```python
from build123d import *

# Parameters (mm, degrees)
F0_W     = 177.8
F0_H     = 137.16
F0_R     = 6.35
F1_DEPTH = 6.35


with BuildPart() as f1:
    # F0 (on Top) → F1 (new body)
    with BuildSketch(Plane.XY):
        with Locations((80.01, 53.34)):
            Rectangle(F0_W, F0_H)
        Circle(F0_R, mode=Mode.SUBTRACT)
        with Locations((17.78, 0)):
            Circle(F0_R, mode=Mode.SUBTRACT)
        with Locations((0, 15.24)):
            Circle(F0_R, mode=Mode.SUBTRACT)
        with Locations((17.78, 15.24)):
            Circle(F0_R, mode=Mode.SUBTRACT)
        with Locations((35.56, 0)):
            Circle(F0_R, mode=Mode.SUBTRACT)
        with Locations((53.34, 0)):
            Circle(F0_R, mode=Mode.SUBTRACT)
        with Locations((71.12, 0)):
            Circle(F0_R, mode=Mode.SUBTRACT)
        with Locations((35.56, 15.24)):
            Circle(F0_R, mode=Mode.SUBTRACT)
        with Locations((53.34, 15.24)):
            Circle(F0_R, mode=Mode.SUBTRACT)
        with Locations((71.12, 15.24)):
            Circle(F0_R, mode=Mode.SUBTRACT)
        with Locations((0, 30.48)):
            Circle(F0_R, mode=Mode.SUBTRACT)
        with Locations((17.78, 30.48)):
            Circle(F0_R, mode=Mode.SUBTRACT)
        with Locations((0, 45.72)):
            Circle(F0_R, mode=Mode.SUBTRACT)
        with Locations((17.78, 45.72)):
            Circle(F0_R, mode=Mode.SUBTRACT)
        with Locations((35.56, 30.48)):
            Circle(F0_R, mode=Mode.SUBTRACT)
        with Locations((53.34, 30.48)):
            Circle(F0_R, mode=Mode.SUBTRACT)
        with Locations((71.12, 30.48)):
            Circle(F0_R, mode=Mode.SUBTRACT)
        with Locations((35.56, 45.72)):
            Circle(F0_R, mode=Mode.SUBTRACT)
        with Locations((53.34, 45.72)):
            Circle(F0_R, mode=Mode.SUBTRACT)
        with Locations((71.12, 45.72)):
            Circle(F0_R, mode=Mode.SUBTRACT)
        with Locations((88.9, 0)):
            Circle(F0_R, mode=Mode.SUBTRACT)
        with Locations((106.68, 0)):
            Circle(F0_R, mode=Mode.SUBTRACT)
        with Locations((124.46, 0)):
            Circle(F0_R, mode=Mode.SUBTRACT)
        with Locations((88.9, 15.24)):
            Circle(F0_R, mode=Mode.SUBTRACT)
        with Locations((106.68, 15.24)):
            Circle(F0_R, mode=Mode.SUBTRACT)
        with Locations((124.46, 15.24)):
            Circle(F0_R, mode=Mode.SUBTRACT)
        with Locations((142.24, 0)):
            Circle(F0_R, mode=Mode.SUBTRACT)
        with Locations((160.02, 0)):
            Circle(F0_R, mode=Mode.SUBTRACT)
        with Locations((142.24, 15.24)):
            Circle(F0_R, mode=Mode.SUBTRACT)
        with Locations((160.02, 15.24)):
            Circle(F0_R, mode=Mode.SUBTRACT)
        with Locations((88.9, 30.48)):
            Circle(F0_R, mode=Mode.SUBTRACT)
        with Locations((106.68, 30.48)):
            Circle(F0_R, mode=Mode.SUBTRACT)
        with Locations((124.46, 30.48)):
            Circle(F0_R, mode=Mode.SUBTRACT)
        with Locations((88.9, 45.72)):
            Circle(F0_R, mode=Mode.SUBTRACT)
        with Locations((106.68, 45.72)):
            Circle(F0_R, mode=Mode.SUBTRACT)
        with Locations((124.46, 45.72)):
            Circle(F0_R, mode=Mode.SUBTRACT)
        with Locations((142.24, 30.48)):
            Circle(F0_R, mode=Mode.SUBTRACT)
        with Locations((160.02, 30.48)):
            Circle(F0_R, mode=Mode.SUBTRACT)
        with Locations((142.24, 45.72)):
            Circle(F0_R, mode=Mode.SUBTRACT)
        with Locations((160.02, 45.72)):
            Circle(F0_R, mode=Mode.SUBTRACT)
        with Locations((0, 60.96)):
            Circle(F0_R, mode=Mode.SUBTRACT)
        with Locations((17.78, 60.96)):
            Circle(F0_R, mode=Mode.SUBTRACT)
        with Locations((35.56, 60.96)):
            Circle(F0_R, mode=Mode.SUBTRACT)
        with Locations((53.34, 60.96)):
            Circle(F0_R, mode=Mode.SUBTRACT)
        with Locations((71.12, 60.96)):
            Circle(F0_R, mode=Mode.SUBTRACT)
        with BuildLine():
            ThreePointArc((8.255, 102.87), (10.114872, 107.360128), (14.605, 109.22))
            Line((14.605, 109.22), (62.865, 109.22))
            ThreePointArc((62.865, 109.22), (67.355128, 107.360128), (69.215, 102.87))
            Line((69.215, 102.87), (69.215, 85.09))
            ThreePointArc((69.215, 85.09), (67.355128, 80.599872), (62.865, 78.74))
            Line((62.865, 78.74), (14.605, 78.74))
            ThreePointArc((14.605, 78.74), (10.114872, 80.599872), (8.255, 85.09))
            Line((8.255, 85.09), (8.255, 102.87))
        make_face(mode=Mode.SUBTRACT)
        with Locations((88.9, 60.96)):
            Circle(F0_R, mode=Mode.SUBTRACT)
        with Locations((106.68, 60.96)):
            Circle(F0_R, mode=Mode.SUBTRACT)
        with Locations((124.46, 60.96)):
            Circle(F0_R, mode=Mode.SUBTRACT)
        with Locations((88.9, 76.2)):
            Circle(F0_R, mode=Mode.SUBTRACT)
        with Locations((106.68, 76.2)):
            Circle(F0_R, mode=Mode.SUBTRACT)
        with Locations((124.46, 76.2)):
            Circle(F0_R, mode=Mode.SUBTRACT)
        with Locations((142.24, 60.96)):
            Circle(F0_R, mode=Mode.SUBTRACT)
        with Locations((160.02, 60.96)):
            Circle(F0_R, mode=Mode.SUBTRACT)
        with Locations((142.24, 76.2)):
            Circle(F0_R, mode=Mode.SUBTRACT)
        with Locations((160.02, 76.2)):
            Circle(F0_R, mode=Mode.SUBTRACT)
        with Locations((88.9, 91.44)):
            Circle(F0_R, mode=Mode.SUBTRACT)
        with Locations((106.68, 91.44)):
            Circle(F0_R, mode=Mode.SUBTRACT)
        with Locations((124.46, 91.44)):
            Circle(F0_R, mode=Mode.SUBTRACT)
        with Locations((88.9, 106.68)):
            Circle(F0_R, mode=Mode.SUBTRACT)
        with Locations((106.68, 106.68)):
            Circle(F0_R, mode=Mode.SUBTRACT)
        with Locations((124.46, 106.68)):
            Circle(F0_R, mode=Mode.SUBTRACT)
        with Locations((142.24, 91.44)):
            Circle(F0_R, mode=Mode.SUBTRACT)
        with Locations((160.02, 91.44)):
            Circle(F0_R, mode=Mode.SUBTRACT)
        with Locations((142.24, 106.68)):
            Circle(F0_R, mode=Mode.SUBTRACT)
        with Locations((160.02, 106.68)):
            Circle(F0_R, mode=Mode.SUBTRACT)
    extrude(amount=F1_DEPTH)


solid = f1.part
```
Build history of the part. All positions in model axes, mm. Round coordinates to 2 decimals unless told otherwise and drop trailing zeros. Order: outer loops, then holes, each group sorted by start corner. A loop starts at its lowest first (then second) coordinate and runs counter-clockwise, first axis right, second up. Notation, with made-up numbers: (70, -34.5) -> (113, -34.5) arc R20 cw to (113, -16.5) -> close; hole circle Ø4 at (-6.5, 4). An arc over 180 degrees is marked (long way). Answer in a Markdown table with one row per item.
1) Pin check, flat tips, straight feed: P1, Ø20.5, axis at x = 142.24, y = 15.24, coming from the -Z side; P2, Ø7.5, axis at x = 88.9, y = 30.48, coming from the +Z side. Stop position of each tip, or through.
Values:
| item | result |
|---|---|
| P1 | z = 0 |
| P2 | through |
2) Wall check: L1, parallel to X at y = 98, z = 5 (3 decimals); L2, parallel to Y at x = 62.5, z = 3.5; L3, parallel to X at y = 74, z = 3.25. Give the ranges that are in metal, low to high.
Values:
| item | result |
|---|---|
| L1 | -8.89 to 8.255, 69.215 to 168.91 |
| L2 | -15.24 to 78.74, 109.22 to 121.92 |
| L3 | -8.89 to 82.94, 94.86 to 100.72, 112.64 to 118.5, 130.42 to 136.28, 148.2 to 154.06, 165.98 to 168.91 |
3) Mould opens along X. For faces 1 (the cylindrical face through (64.776, 61.239, 3.131)), 2 (the flat face through (-8.89, 52, 3)) say: released by +X, released by -X, zero draft, split by the parting line, or undercut.
Values:
| item | result |
|---|---|
| face 1 | undercut |
| face 2 | released by -X |
4) Band-saw the part on C-C on y = 0. Give the number of separate pieces and of enclosed holes in the cut face, and give its area (3 significant figures).
Values:
| item | result |
|---|---|
| separate pieces | 11 |
| enclosed holes | 0 |
| area | 323 mm2 |
5) Band-saw the part on B-B on y = 106.68. Give the cut face in (x, z) (3 decimals).
Values:
| item | result |
|---|---|
| outline | (-8.89, 0) -> (9.525, 0) -> (9.525, 6.35) -> (-8.89, 6.35) -> close; (67.945, 0) -> (82.55, 0) -> (82.55, 6.35) -> (67.945, 6.35) -> close; (95.25, 0) -> (100.33, 0) -> (100.33, 6.35) -> (95.25, 6.35) -> close; (113.03, 0) -> (118.11, 0) -> (118.11, 6.35) -> (113.03, 6.35) -> close; (130.81, 0) -> (135.89, 0) -> (135.89, 6.35) -> (130.81, 6.35) -> close; (148.59, 0) -> (153.67, 0) -> (153.67, 6.35) -> (148.59, 6.35) -> close; (166.37, 0) -> (168.91, 0) -> (168.91, 6.35) -> (166.37, 6.35) -> close |
6) Band-saw the part on A-A on x = 71.12. Give the cut face in (y, z).
Values:
| item | result |
|---|---|
| outline | (-15.24, 0) -> (-6.35, 0) -> (-6.35, 6.35) -> (-15.24, 6.35) -> close; (6.35, 0) -> (8.89, 0) -> (8.89, 6.35) -> (6.35, 6.35) -> close; (21.59, 0) -> (24.13, 0) -> (24.13, 6.35) -> (21.59, 6.35) -> close; (36.83, 0) -> (39.37, 0) -> (39.37, 6.35) -> (36.83, 6.35) -> close; (52.07, 0) -> (54.61, 0) -> (54.61, 6.35) -> (52.07, 6.35) -> close; (67.31, 0) -> (121.92, 0) -> (121.92, 6.35) -> (67.31, 6.35) -> close |
